Verification items for this drawing (mm, ordinates from the low corner). Round coordinates to 2 decimals unless told otherwise and drop trailing zeros. Loops run counter-clockwise (first coordinate to the right, second up) from the corner with the lowest first, then second, coordinate; pieces in that order, holes last. Notation, with made-up numbers: M -22.5,77.25 L 35.5,77.25 A25 ccw 35.5,113.25 Z; hole C 42,78 d9. An arc over 180 degrees is marked long. Answer as CSV lines item,"result".
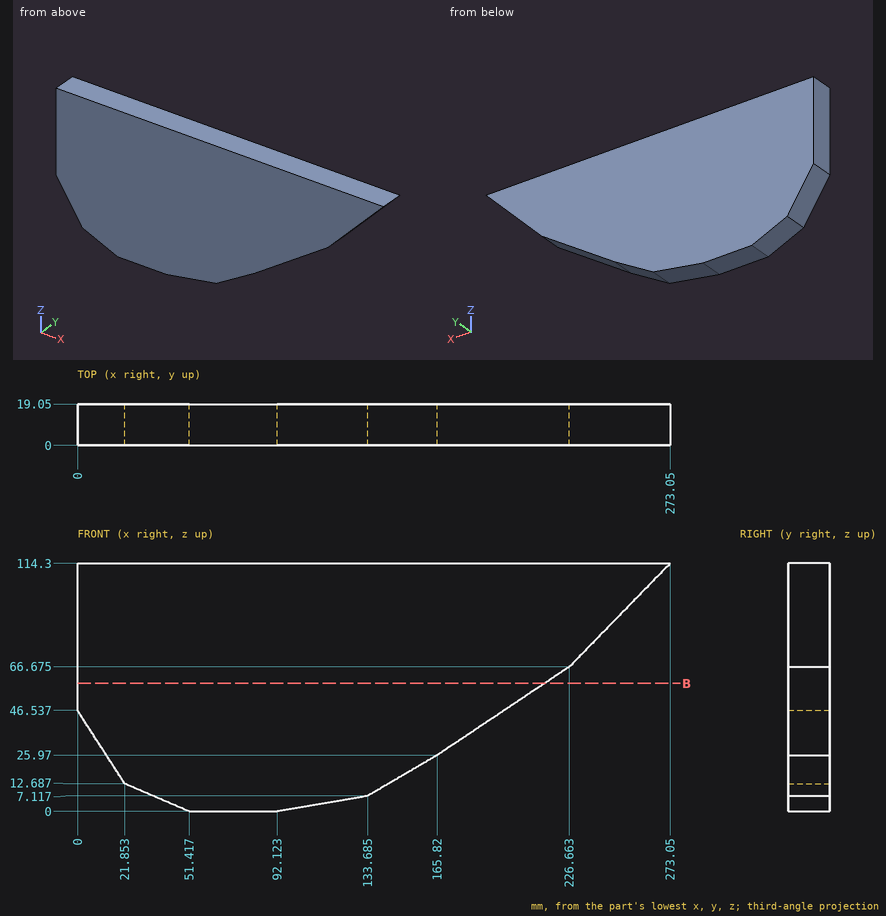
1) Material ranges on probe 1 along X at (y, z) = (15.5, 15) (1 decimal); probe 2 along X at (y, z) = (16.25, 57.5); probe 3 along Z at (x, y) = (210, 3.25) (1 decimal), recorded low to high.
Here are the results:
probe 1,"x = 20.4 to 147.1"
probe 2,"x = 0 to 212.95"
probe 3,"z = 55.5 to 114.3"
2) Go/stop test with flat-tipped pins: pin 1 (8 mm diameter, centred on x = 35, z = 76, fed in from -Y); pin 2 (3 mm diameter, centred on y = 3, z = 43, fed in from -X) (1 decimal); pin 3 (5 mm diameter, centred on y = 16, z = 21.5, fed in from -X). Record where each tip stops, or that it passes through.
Here are the results:
pin 1,"stops at y = 0"
pin 2,"stops at x = 1.3"
pin 3,"stops at x = 14.55"
3) Section check B-B (z = 59). Record the cut outline in (x, y), plus the area to 3 significant figures.
Here are the results:
outline,"M 0,0 L 215.19,0 L 215.19,19.05 L 0,19.05 Z"
area,"4,100 mm^2"
